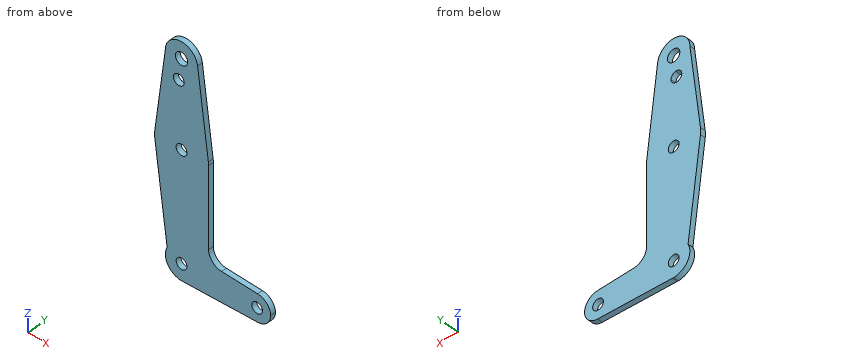
```python
from build123d import *

# Parameters (mm, degrees)
F0_R     = 3.639412
F0_R_2   = 3.175
F1_DEPTH = 3.048


with BuildPart() as f1:
    # F0 (on Front) → F1 (new body)
    with BuildSketch(Plane.XZ):
        with BuildLine():
            ThreePointArc((9.450293, 115.490625), (9.506305, 114.896483), (9.525, 114.3))
            ThreePointArc((9.525, 114.3), (6.300195, 107.15625), (-1.190625, 104.849707))
            ThreePointArc((-1.190625, 104.849707), (-7.14375, 107.999805), (-9.525, 114.3))
            Line((-9.525, 114.3), (-15.747457, 65.508289))
            ThreePointArc((-15.747457, 65.508289), (0.012053, 79.374995), (15.750488, 65.484375))
            Line((15.750488, 65.484375), (9.450293, 115.490625))
        make_face()
        with BuildLine():
            ThreePointArc((1.5875, 101.699609), (-3.96875, 99.599544), (-1.190625, 104.849707))
            ThreePointArc((-1.190625, 104.849707), (0.79375, 103.799675), (1.5875, 101.699609))
        make_face(mode=Mode.SUBTRACT)
        with BuildLine():
            ThreePointArc((-1.190625, 104.849707), (6.300195, 107.15625), (9.525, 114.3))
            ThreePointArc((9.525, 114.3), (9.506305, 114.896483), (9.450293, 115.490625))
            ThreePointArc((9.450293, 115.490625), (-0.596483, 123.806305), (-9.525, 114.3))
            ThreePointArc((-9.525, 114.3), (-7.14375, 107.999805), (-1.190625, 104.849707))
        make_face()
        with Locations((0, 114.3)):
            Circle(F0_R, mode=Mode.SUBTRACT)
        with BuildLine():
            ThreePointArc((15.875, 63.5), (15.843841, 64.494139), (15.750488, 65.484375))
            ThreePointArc((15.750488, 65.484375), (0.012053, 79.374995), (-15.747457, 65.508289))
            ThreePointArc((-15.747457, 65.508289), (-15.875, 63.5), (-15.747457, 61.491711))
            ThreePointArc((-15.747457, 61.491711), (1.006168, 47.656918), (15.875, 63.5))
        make_face()
        with Locations((0, 63.5)):
            Circle(F0_R_2, mode=Mode.SUBTRACT)
        with BuildLine():
            Line((15.875, 16.632032), (15.875, 63.5))
            ThreePointArc((15.875, 63.5), (1.006168, 47.656918), (-15.747457, 61.491711))
            Line((-15.747457, 61.491711), (-8.462807, 4.371101))
            ThreePointArc((-8.462807, 4.371101), (2.249154, 9.255643), (9.525, 0))
            ThreePointArc((9.525, 0), (6.970557, -6.491299), (0.677344, -9.500886))
            Line((0.677344, -9.500886), (44.732405, -7.932475))
            ThreePointArc((44.732405, -7.932475), (36.5125, 0), (44.732405, 7.932475))
            Line((44.732405, 7.932475), (23.542343, 8.686865))
            ThreePointArc((23.542343, 8.686865), (18.104429, 11.111302), (15.875, 16.632032))
        make_face()
        with BuildLine():
            ThreePointArc((9.525, 0), (2.249154, 9.255643), (-8.462807, 4.371101))
            ThreePointArc((-8.462807, 4.371101), (-8.13512, -4.954336), (0, -9.525))
            Line((0, -9.525), (0.677344, -9.500886))
            ThreePointArc((0.677344, -9.500886), (6.970557, -6.491299), (9.525, 0))
        make_face()
        Circle(F0_R_2, mode=Mode.SUBTRACT)
        with BuildLine():
            ThreePointArc((52.3875, 0), (50.161633, 5.51191), (44.732405, 7.932475))
            ThreePointArc((44.732405, 7.932475), (36.5125, 0), (44.732405, -7.932475))
            ThreePointArc((44.732405, -7.932475), (50.161633, -5.51191), (52.3875, 0))
        make_face()
        with Locations((44.45, 0)):
            Circle(F0_R_2, mode=Mode.SUBTRACT)
    extrude(amount=F1_DEPTH)


solid = f1.part
```
The listing builds one solid part. Answer for the finished solid, in the listing's coordinates (mm). Coordinates: 2 decimals unless noted, no trailing zeros. Loops run counter-clockwise (first coordinate to the right, second up) from the corner with the lowest first, then second, coordinate; pieces in that order, holes last. Notation, with made-up numbers: M -17,25.25 L 32,25.25 A9 ccw 32,29.25 Z; hole C 80,18.25 d5. An arc over 180 degrees is marked long. Answer as a JSON object with one key per item and string values. Group by question number.
Item 1: Consider L1, parallel to Z at x = 44.45, y = -0.9 (3 decimals); L2, parallel to Z at x = 0, y = -1.8 (3 decimals); L3, parallel to X at y = -1.9, z = 116. Determine where each line is inside the solid, lowest interval first.
Item 2: Section B-B (z = 12) is taken. Write down the section's boundary in (x, y).
Item 3: Each of these flat-tipped pins is pushed along its axis until it touches: P1, Ø5, axis at x = 44.45, z = 0, coming from the +Y side; P2, Ø0.9, axis at y = -1, z = 32, coming from the +X side (3 decimals); P3, Ø1, axis at y = -2, z = 33, coming from the -X side. Where does it stop, or does it pass through?
Item 4: Section A-A (y = -2.25) is taken. Give the number of separate pieces and of enclosed holes in the cut face, and give its area (3 significant figures).
Solved:
{
 "1": {"L1": "z = -7.943 to -3.175, 3.175 to 7.943", "L2": "z = -9.525 to -3.175, 3.175 to 60.325, 66.675 to 98.95, 104.449 to 110.661, 117.939 to 123.825", "L3": "x = -9.37 to -3.22, 3.22 to 9.37"},
 "2": {"outline": "M -9.44,-3.05 L 17.36,-3.05 L 17.36,0 L -9.44,0 Z"},
 "3": {"P1": "passes through", "P2": "stops at x = 15.875", "P3": "stops at x = -12.18"},
 "4": {"separate pieces": "1", "enclosed holes": "5", "area": "3,860 mm2"}
}
